Input: part model. Units: mm. Frame: model coordinates. A direction names the side the tool comes from. Coordinates: 2 decimals unless noted, no trailing zeros. Loops run counter-clockwise (first coordinate to the right, second up) from the corner with the lowest first, then second, coordinate; pieces in that order, holes last. Notation, with made-up numbers: (81, -1) - (111, -1) arc R22 ccw to (111, 25) - close; hole circle Ø4 at (67, 89). An arc over 180 degrees is marked (long way). Answer as CSV lines item,"result". Start each with the question number.
```python
from build123d import *

# Parameters (mm, degrees)
SKETCH1_R           = 3
BOSS_EXTRUDE1_DEPTH = 2.5
CUT_EXTRUDE1_DEPTH  = 6
CUT_EXTRUDE2_DEPTH  = 25.4


with BuildPart() as part:
    # Sketch1 → Boss-Extrude1 (new body, symmetric)
    with BuildSketch(Plane.XY):
        Polygon((20.32, 12.7), (20.32, -12.7), (-17.78, -12.7), (-62.5670531, 241.3), (-37.552936173, 245.710663713), (3.533130632, 12.7), align=None)
        Circle(SKETCH1_R, mode=Mode.SUBTRACT)
    extrude(amount=BOSS_EXTRUDE1_DEPTH, both=True)

    # Sketch2 → Cut-Extrude1 (cut, through all)
    with BuildSketch(Plane.XY.offset(2.5)):
        Polygon((-37.552936173, 245.710663713), (3.533130632, 12.7), (-4.204420151, 12.7), (-45.057171251, 244.387464599), align=None)
    extrude(amount=-CUT_EXTRUDE1_DEPTH, mode=Mode.SUBTRACT)

    # Sketch3 → Cut-Extrude2 (cut, symmetric)
    with BuildSketch(Plane.XY):
        Polygon((-42.057332667, 167.540909253), (-39.102909408, 168.061853786), (-25.87091827, 93.019503007), (-28.825341529, 92.498558474), align=None)
    extrude(amount=CUT_EXTRUDE2_DEPTH, both=True, mode=Mode.SUBTRACT)


solid = part.part
```
Item 1: Material intervals for probe 1 along Y at (x, z) = (0, 1.4); probe 2 along Y at (x, z) = (-1, 0.3); probe 3 along X at (y, z) = (143, -0.1), sorted ascending.
Item 2: Set-up query: faces 1 (the flat face through (-32.58, 131.07, 0.04)), 2 (the flat face through (8, 12.7, 0)), 3 (the flat face through (-24, 97, -2.5)). Return all of +Z, -Z, +X, -X, +Y, -Y with unobstructed straight access to the full face (end or side cutting, diameter ignored); none if empty.
Item 3: Section query A-A, the plane x = 0. Output: boundary loops of the cut face in (y, z).
Item 4: Contact query for flat-ended pins moving along their axis: P1, Ø3.5, axis at x = 0, y = 0, coming from the -Z side; P2, Ø3, axis at y = 29, z = 0, coming from the +X side; P3, Ø2, axis at y = 82.5, z = 0.5, coming from the -X side; P4, Ø1.5, axis at x = 13.5, z = 0.5, coming from the +Y side. Output: stop coordinate, or through.
Item 5: Draft query along Y for faces 4 (the flat face through (2, -12.7, 0)), 5 (the flat face through (-24, 97, 2.5)), 6 (the cylindrical face through (-3, 0, 0)). Return one class per face: pulls with the +Y half, pulls with the -Y half, needs draft (parallel to the pull), parting line crosses it, or undercut.
Item 6: Section query B-B, the plane z = 0.7. Output: boundary loops of the cut face in (x, y).
Item 7: Section query C-C, the plane y = 0. Output: boundary loops of the cut face in (x, z).
Item 8: Section query D-D, the plane x = 12. Output: boundary loops of the cut face in (y, z).
Response values:
1,probe 1,"y = -12.7 to -3, 3 to 12.7"
1,probe 2,"y = -12.7 to -2.83, 2.83 to 12.7"
1,probe 3,"x = -45.23 to -37.73, -34.68 to -27.18"
2,face 1,"+Z, -Z"
2,face 2,"+Z, -Z, +X, +Y"
2,face 3,"-Z, +X, -X, +Y, -Y"
3,outline,"(-12.7, -2.5) - (-3, -2.5) - (-3, 2.5) - (-12.7, 2.5) - close; (3, -2.5) - (12.7, -2.5) - (12.7, 2.5) - (3, 2.5) - close"
4,P1,"passes through"
4,P2,"stops at x = -6.81"
4,P3,"stops at x = -34.74"
4,P4,"stops at y = 12.7"
5,face 4,"pulls with the -Y half"
5,face 5,"needs draft"
5,face 6,"undercut"
6,outline,"(-62.57, 241.3) - (-17.78, -12.7) - (20.32, -12.7) - (20.32, 12.7) - (-4.2, 12.7) - (-45.06, 244.39) - close; hole (-42.06, 167.54) - (-28.83, 92.5) - (-25.87, 93.02) - (-39.1, 168.06) - close; hole circle Ø6 at (0, 0)"
7,outline,"(-20.02, -2.5) - (-3, -2.5) - (-3, 2.5) - (-20.02, 2.5) - close; (3, -2.5) - (20.32, -2.5) - (20.32, 2.5) - (3, 2.5) - close"
8,outline,"(-12.7, -2.5) - (12.7, -2.5) - (12.7, 2.5) - (-12.7, 2.5) - close"
